Geometry: final body of the model. Coordinates: model frame, mm. A direction names the side the tool comes from. Round coordinates to 2 decimals unless told otherwise and drop trailing zeros. Write each loop counter-clockwise with the first axis right and the second up, starting at its lowest first coordinate (ties: lowest second). Pieces come first, ordered by that corner, then holes. Notation, with made-up numbers: M 3.5,33 L 12.5,33 A15 ccw 12.5,59 Z; hole C 39.25,-27.5 d8. An arc over 180 degrees is marked long. Put each result on its own line as item: value. Start each with the question number.
Solid Edge part; units mm, degrees
sketch "Sketch1" plane through (0, 0, 0) normal (1, 0, 0) x (0, 1, 0)
  line L0 (-34.4663, 68.439) -> (-20.6663, 68.439)
  line L1 (-20.6663, 74.439) -> (-20.6663, 68.439)
  line L2 (-20.6663, 74.439) -> (-34.4663, 74.439)
  line L3 (-34.4663, 74.439) -> (-34.4663, 68.439)
  line L4 (-15.0663, 64.689) -> (-15.0663, 77.689)
  line L5 (-15.0663, 77.689) -> (-40.0663, 77.689)
  line L6 (-40.0663, 77.689) -> (-40.0663, 64.689)
  line L7 (-40.0663, 64.689) -> (-15.0663, 64.689)
extrude "Protrusion1" add sketch "Sketch1" against normal blind 20
sketch "Sketch2" plane through (-10, -27.5663, 77.689) normal (0, 0, 1) x (1, 0, 0)
  line L0 (3.5, 12.5) -> (3.5, -12.5)
  line L1 (3.5, -12.5) -> (10, -12.5)
  line L2 (10, -12.5) -> (10, 12.5)
  line L3 (10, 12.5) -> (3.5, 12.5)
extrude "Cutout1" cut sketch "Sketch2" against normal up to vertex (9.25 mm away)
sketch "Sketch3" plane through (-10, -27.5663, 77.689) normal (0, 0, 1) x (1, 0, 0)
  circle A0 centre (6.75, -9.625) radius 1.2
  circle A1 centre (6.75, 9.625) radius 1.2
extrude "Cutout2" cut sketch "Sketch3" against normal up to next
1) Section A-A, the plane x = -3.25. Output: boundary loops of the cut face in (y, z).
2) Section D-D, the plane x = -13.75. Output: boundary loops of the cut face in (y, z).
3) Draft query along Y for faces 3 (the face through (-8, -27, 68.439)), 4 (the face through (-12, -40.066, 71)), 5 (the face through (-6.5, -27, 75)), 6 (the face through (-2.7, -19.01, 66.59)). Return one class per face: +Y half, -Y half, draft (parallel to the pull), parting line (faces both ways), or undercut.
4) Ray query, probe 1 along Y at (x, z) = (-3.25, 66.35); probe 2 along Y at (x, z) = (-9.5, 73.75); probe 3 along Z at (x, y) = (-15, -21.5). Return the intervals inside material, ascending.
5) Access query for faces 1 (the face through (0, -28, 67)), 2 (the face through (-13, -27, 74.439)). Directions: +Z, -Z, +X, -X, +Y, -Y. A direction counts if a zero-diameter tool reaches every point of the face in a straight line with its end or side. Return the directions, or none.
6) First-contact query: pin 1 (2 mm diameter, centred on x = -3.25, y = -17.94, fed in from -Z); pin 2 (3 mm diameter, centred on x = -3.25, y = -37.19, fed in from +Z); pin 3 (4 mm diameter, centred on y = -18.5, z = 76, fed in from +X). Flat tips, straight axial feed; report the tip coordinate or a pass-through.
7) Section B-B, the plane z = 71.25. Output: boundary loops of the cut face in (x, y).
8) Section C-C, the plane y = -27.5. Output: boundary loops of the cut face in (x, z), and give its area (3 significant figures).
Solved:
1. outline: M -40.07,64.69 L -38.39,64.69 L -38.39,68.44 L -40.07,68.44 Z; M -35.99,64.69 L -19.14,64.69 L -19.14,68.44 L -35.99,68.44 Z; M -16.74,64.69 L -15.07,64.69 L -15.07,68.44 L -16.74,68.44 Z
2. outline: M -40.07,64.69 L -15.07,64.69 L -15.07,77.69 L -40.07,77.69 Z; hole M -34.47,68.44 L -20.67,68.44 L -20.67,74.44 L -34.47,74.44 Z
3. face 3: undercut
3. face 4: -Y half
3. face 5: draft
3. face 6: undercut
4. probe 1: y = -40.07 to -38.39, -35.99 to -19.14, -16.74 to -15.07
4. probe 2: y = -40.07 to -34.47, -20.67 to -15.07
4. probe 3: z = 64.69 to 68.44, 74.44 to 77.69
5. face 1: +Z, -Z, +X, +Y, -Y
5. face 2: +X, -X
6. pin 1: passes through
6. pin 2: stops at z = 68.44
6. pin 3: stops at x = -6.5
7. outline: M -20,-40.07 L -6.5,-40.07 L -6.5,-34.47 L -20,-34.47 Z; M -20,-20.67 L -6.5,-20.67 L -6.5,-15.07 L -20,-15.07 Z
8. outline: M -20,64.69 L 0,64.69 L 0,68.44 L -20,68.44 Z; M -20,74.44 L -6.5,74.44 L -6.5,77.69 L -20,77.69 Z
8. area: 119 mm2
